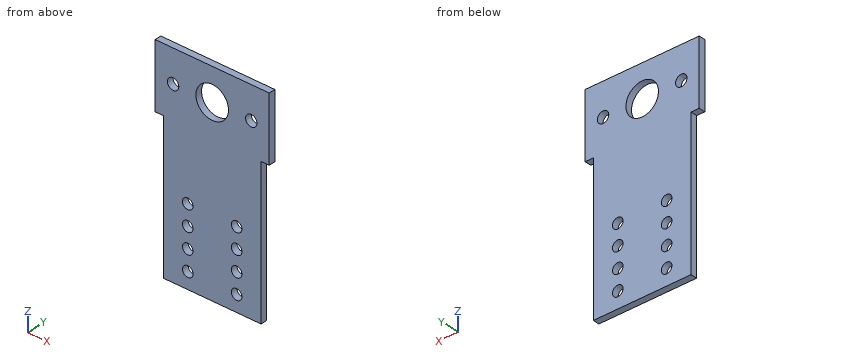
```python
from build123d import *

# Parameters (mm, degrees)
SKETCH1_W           = 60
SKETCH1_H           = 130
BOSS_EXTRUDE1_DEPTH = 4
SKETCH2_W           = 70
SKETCH2_H           = 40
BOSS_EXTRUDE2_DEPTH = 4
SKETCH3_R           = 3.5
SKETCH3_R_2         = 10
CUT_EXTRUDE1_DEPTH  = 5
CUT_EXTRUDE2_START  = -5
SKETCH4_R           = 3.25
CUT_EXTRUDE2_DEPTH  = 6
LPATTERN1_COUNT     = 4
LPATTERN1_PITCH     = 12.5


with BuildPart() as part:
    # Sketch1 → Boss-Extrude1 (new body)
    with BuildSketch(Plane(origin=(0, 0, 0), x_dir=(1, 0, 0), z_dir=(0, 1, 0))):
        Rectangle(SKETCH1_W, SKETCH1_H)
    extrude(amount=BOSS_EXTRUDE1_DEPTH)

    # Sketch2 → Boss-Extrude2 (add)
    with BuildSketch(Plane(origin=(0, 0, 0), x_dir=(1, 0, 0), z_dir=(0, 1, 0))):
        with Locations((0, -45)):
            Rectangle(SKETCH2_W, SKETCH2_H)
    extrude(amount=BOSS_EXTRUDE2_DEPTH)

    # Sketch3 → Cut-Extrude1 (cut, through all)
    with BuildSketch(Plane(origin=(0, 4, 0), x_dir=(1, 0, 0), z_dir=(0, 1, 0))):
        with Locations((24, -45)):
            Circle(SKETCH3_R)
        with Locations((-24, -45)):
            Circle(SKETCH3_R)
        with Locations((0, -45)):
            Circle(SKETCH3_R_2)
    extrude(amount=-CUT_EXTRUDE1_DEPTH, mode=Mode.SUBTRACT)

    # Sketch4 → Cut-Extrude2 (cut)
    with BuildSketch(Plane(origin=(0, 4, 0), x_dir=(1, 0, 0), z_dir=(0, 1, 0)).offset(CUT_EXTRUDE2_START)):
        with Locations((15, 55)):
            Circle(SKETCH4_R)
        with Locations((-15, 55)):
            Circle(SKETCH4_R)
    cut_extrude2 = extrude(amount=CUT_EXTRUDE2_DEPTH, mode=Mode.SUBTRACT)

    # LPattern1: Cut-Extrude2 ×4
    with Locations(*[(0, 0, i * LPATTERN1_PITCH) for i in range(1, LPATTERN1_COUNT)]):
        add(cut_extrude2, mode=Mode.SUBTRACT)


solid = part.part
```
Geometry check sheet. Reference: the model listing, model coordinates, mm. Coordinates: 2 decimals unless noted, no trailing zeros. Write each loop counter-clockwise with the first axis right and the second up, starting at its lowest first coordinate (ties: lowest second). Pieces come first, ordered by that corner, then holes. Notation, with made-up numbers: M 42,18 L 89,18 A32 ccw 89,56 Z; hole C 73,-14.5 d7. An arc over 180 degrees is marked long. Use one line per item in the form item = value. Start each with the question number.
1) Section check D-D on y = 1.05. State how many separate pieces and enclosed holes the cut face has, and give its area (3 significant figures).
2) Section check A-A on x = 24. Enter the section's corners in (y, z), and give its area (3 significant figures).
3) Thickness scan on probe 1 along Z at (x, y) = (-15, 2.65); probe 2 along X at (y, z) = (3.15, 45); probe 3 along Z at (x, y) = (24, 1.7). Record the ranges inside material, lowest first. Write a range as from..to.
4) Section check C-C on z = -55. Enter the section's corners in (x, y), and give its area (3 significant figures).
5) Section check B-B on x = 15. Enter the section's corners in (y, z), and give its area (3 significant figures).
6) Go/stop test with flat-tipped pins: pin 1 Ø2 at (y, z) = (2.5, -39.5) entering from +X; pin 2 Ø1.2 at (x, y) = (-33, 2) entering from -Z; pin 3 Ø2 at (y, z) = (1.5, -22) entering from -X. Record where each tip stops, or that it passes through.
Responses:
q1.separate_pieces = 1
q1.enclosed_holes = 11
q1.area = 7,540 mm2
q2.outline = M 0,-65 L 4,-65 L 4,41.5 L 0,41.5 Z; M 0,48.5 L 4,48.5 L 4,65 L 0,65 Z
q2.area = 492 mm2
q3.probe_1 = -65..-58.25, -51.75..-45.75, -39.25..-33.25, -26.75..-20.75, -14.25..65
q3.probe_2 = -35..-27.5, -20.5..-10, 10..20.5, 27.5..35
q3.probe_3 = -65..41.5, 48.5..65
q4.outline = M -30,0 L -18.25,0 L -18.25,4 L -30,4 Z; M -11.75,0 L 11.75,0 L 11.75,4 L -11.75,4 Z; M 18.25,0 L 30,0 L 30,4 L 18.25,4 Z
q4.area = 188 mm2
q5.outline = M 0,-65 L 4,-65 L 4,-58.25 L 0,-58.25 Z; M 0,-51.75 L 4,-51.75 L 4,-45.75 L 0,-45.75 Z; M 0,-39.25 L 4,-39.25 L 4,-33.25 L 0,-33.25 Z; M 0,-26.75 L 4,-26.75 L 4,-20.75 L 0,-20.75 Z; M 0,-14.25 L 4,-14.25 L 4,65 L 0,65 Z
q5.area = 416 mm2
q6.pin_1 = 30
q6.pin_2 = 25
q6.pin_3 = -30
